from build123d import *

# Parameters (mm, degrees)
SKETCH1_W               = 3
SKETCH1_H               = 42.1
SKETCH1_H_2             = 4
BOSS_EXTRUDE1_DEPTH     = 12
SKETCH3_W               = 45.1
SKETCH3_H               = 17.9
SKETCH3_R               = 1.5
BOSS_EXTRUDE2_DEPTH     = 3
SKETCH5_W               = 17.9
SKETCH5_H               = 45.1
BOSS_EXTRUDE4_DEPTH     = 4.5
CUT_EXTRUDE4_DEPTH      = 54.638254019
CUT_EXTRUDE5_DEPTH      = 54.638254019
CUT_EXTRUDE5_DEPTH_BACK = 7.5
SKETCH7_W               = 17.9
SKETCH7_H               = 45.1


with BuildPart() as part:
    # Sketch1 → Boss-Extrude1 (new body)
    with BuildSketch(Plane.YZ):
        Polygon((-5.95, 3.8), (5.95, 3.8), (8.95, 3.8), (8.95, 6.8), (-8.95, 6.8), (-8.95, 3.8), align=None)
        with Locations((-7.45, -17.25)):
            Rectangle(SKETCH1_W, SKETCH1_H)
        with Locations((7.45, -17.25)):
            Rectangle(SKETCH1_W, SKETCH1_H)
        with Locations((0, -32.3)):
            Rectangle(SKETCH1_W, SKETCH1_H_2)
    extrude(amount=BOSS_EXTRUDE1_DEPTH)

    # Sketch3 → Boss-Extrude2 (add)
    with BuildSketch(Plane.ZY):
        with Locations((-15.75, 0)):
            Rectangle(SKETCH3_W, SKETCH3_H)
        Circle(SKETCH3_R, mode=Mode.SUBTRACT)
    extrude(amount=BOSS_EXTRUDE2_DEPTH)

    # Sketch5 → Boss-Extrude4 (add)
    with BuildSketch(Plane(origin=(-3, 0, 0), x_dir=(0, -1, 0), z_dir=(-1, 0, 0))):
        Polygon((-13.95, 21.583539772), (-13.95, -49.572772711), (13.95, -49.572772711), (13.95, 20.927227289), (13.95, 30.427227289), (-13.95, 30.427227289), align=None)
        with Locations((0, -15.75)):
            Rectangle(SKETCH5_W, SKETCH5_H, mode=Mode.SUBTRACT)
    extrude(amount=-BOSS_EXTRUDE4_DEPTH)

    # Sketch6 → Cut-Extrude4 (cut, symmetric)
    with BuildSketch(Plane(origin=(-3, 0, 0), x_dir=(0, -1, 0), z_dir=(-1, 0, 0))):
        with BuildLine():
            Line((-8.95, -4.430558852), (-13.95, -4.430558852))
            ThreePointArc((-13.95, -4.430558852), (-10.365862707, 0.702047669), (-8.95, 6.8))
            Line((-8.95, 6.8), (-13.95, 6.8))
            ThreePointArc((-13.95, 6.8), (-4.216827043, 16.985131712), (0, 30.427227289))
            Line((0, 30.427227289), (0, 38.207310194))
            Line((0, 38.207310194), (-27.495186948, 38.207310194))
            Line((-27.495186948, 38.207310194), (-27.495186948, -49.572772711))
            Line((-27.495186948, -49.572772711), (-5.95, -49.572772711))
            Line((-5.95, -49.572772711), (-5.95, -38.463062756))
            Line((-5.95, -38.463062756), (-13.95, -38.463062756))
            ThreePointArc((-13.95, -38.463062756), (-10.621066319, -33.1423359), (-8.95, -27.092586229))
            Line((-8.95, -27.092586229), (-13.95, -27.092586229))
            ThreePointArc((-13.95, -27.092586229), (-10.764093377, -21.676860063), (-8.95, -15.661117704))
            Line((-8.95, -15.661117704), (-13.95, -15.661117704))
            ThreePointArc((-13.95, -15.661117704), (-10.365862707, -10.528511183), (-8.95, -4.430558852))
        make_face()
    cut_extrude4 = extrude(amount=CUT_EXTRUDE4_DEPTH, both=True, mode=Mode.SUBTRACT)

    # Mirror1: Cut-Extrude4 across plane
    add(cut_extrude4.mirror(Plane.ZX), mode=Mode.SUBTRACT)

    # Sketch7 → Cut-Extrude5 (cut, two sides: drawn at the far end of the back side and taken through both)
    with BuildSketch(Plane.YZ.offset(12).offset(-CUT_EXTRUDE5_DEPTH_BACK)):
        with Locations((0, -15.75)):
            Rectangle(SKETCH7_W, SKETCH7_H)
    extrude(amount=CUT_EXTRUDE5_DEPTH + CUT_EXTRUDE5_DEPTH_BACK, mode=Mode.SUBTRACT)


solid = part.part
For this review, take the finished solid that the model builds, in its own axes (mm). A direction names the side the tool comes from. Coordinates: 2 decimals unless noted, no trailing zeros. Order: outer loops, then holes, each group sorted by start corner. A loop starts at its lowest first (then second) coordinate and runs counter-clockwise, first axis right, second up. Notation, with made-up numbers: (-39, -26) - (14, -26) arc R22 cw to (14, -15) - close; hole circle Ø3 at (-5, 25.25). An arc over 180 degrees is marked (long way). Use one line per item in the form item = value.
Q1. Consider section C-C (z = 0). Give the boundary of the cut face in (x, y), then the cut area to 3 significant figures.
Checked values:
outline = (-3, -10.7) - (1.5, -10.7) - (1.5, -8.95) - (4.5, -8.95) - (4.5, -5.95) - (0, -5.95) - (0, -1.5) - (-3, -1.5) - close; (-3, 1.5) - (0, 1.5) - (0, 5.95) - (4.5, 5.95) - (4.5, 8.95) - (1.5, 8.95) - (1.5, 10.7) - (-3, 10.7) - close
area = 87.4 mm2
Q2. Consider section A-A (x = 3). Give the boundary of the cut face in (y, z), then the cut area to 3 significant figures.
Checked values:
outline = (-8.95, -38.3) - (-5.95, -38.3) - (-5.95, 3.8) - (5.95, 3.8) - (5.95, -38.3) - (8.95, -38.3) - (8.95, 6.8) - (-8.95, 6.8) - close; (-1.5, -34.3) - (1.5, -34.3) - (1.5, -30.3) - (-1.5, -30.3) - close
area = 318 mm2
Q3. For probe 1 along Y at (x, z) = (4, -2.5); probe 2 along X at (y, z) = (-4.25, -38); probe 3 along Z at (x, y) = (-1.5, -12), list the stretches that pass through material, from the lowest coordinate up. Write a range as from..to.
Checked values:
probe_1 = -8.95..-5.95, 5.95..8.95
probe_2 = -3..0
probe_3 = -38.46..-35.77, -27.09..-24.14, -15.66..-13.39, -4.43..-2.16, 6.8..8.18
Q4. Consider section B-B (y = 12.25). Give the boundary of the cut face in (x, z).
Checked values:
outline = (-3, -38.46) - (1.5, -38.46) - (1.5, -36.17) - (-3, -36.17) - close; (-3, -27.09) - (1.5, -27.09) - (1.5, -24.57) - (-3, -24.57) - close; (-3, -15.66) - (1.5, -15.66) - (1.5, -13.73) - (-3, -13.73) - close; (-3, -4.43) - (1.5, -4.43) - (1.5, -2.5) - (-3, -2.5) - close; (-3, 6.8) - (1.5, 6.8) - (1.5, 7.99) - (-3, 7.99) - close
Q5. For faces 4 (the flat face through (-1, -10, -38.463)), 5 (the flat face through (-1, 5.95, -44)), 6 (the flat face through (1.5, 11, -1)), 7 (the flat face through (-1, 11, -15.661)), list the 3-axis set-ups (+Z, -Z, +X, -X, +Y, -Y) from which the entire face can be reached by the end or side of a thin tool; tool diameter is ignored.
Checked values:
face_4 = -Z, +X, -X, -Y
face_5 = -Z, +X, -X, +Y
face_6 = +Z, -Z, +X, +Y
face_7 = +X, -X, +Y
Q6. Consider section D-D (y = 0.75). Give the boundary of the cut face in (x, z).
Checked values:
outline = (-3, -49.57) - (1.5, -49.57) - (1.5, -38.3) - (0, -38.3) - (0, -34.3) - (4.5, -34.3) - (4.5, -30.3) - (0, -30.3) - (0, -1.3) - (-3, -1.3) - close; (-3, 1.3) - (0, 1.3) - (0, 3.8) - (4.5, 3.8) - (4.5, 6.8) - (1.5, 6.8) - (1.5, 25.59) - (-3, 25.59) - close
Q7. Draft analysis for pull direction Z (two halves, no side actions). For faces 1 (the flat face through (3, 0, 6.8)), 2 (the flat face through (2, 0, 3.8)), 3 (the flat face through (1.5, 0, -42)), state which applies: +Z half, -Z half, draft (parallel to the pull), parting line (faces both ways), or undercut.
Checked values:
face_1 = +Z half
face_2 = undercut
face_3 = draft
Q8. For P1, Ø3.5, axis at x = 0.5, y = 11, coming from the -Z side; P2, Ø1.5, axis at y = 11, z = -23.5, coming from the +X side; P3, Ø3.5, axis at y = 0, z = 0, coming from the +X side, all flat-tipped, find the tip position at first contact; note any pin that passes through.
Checked values:
P1 = -38.46
P2 = 1.5
P3 = 0
